CAD build for the part. Positions are in the model's coordinates, mm. A direction names the side the tool comes from. Coordinates: 2 decimals unless noted, no trailing zeros. Loops run counter-clockwise (first coordinate to the right, second up) from the corner with the lowest first, then second, coordinate; pieces in that order, holes last. Notation, with made-up numbers: (-5, -34.75) -> (47, -34.75) arc R32 ccw to (47, -6.75) -> close; hole circle Ø8 at (36.25, -26.5). An arc over 180 degrees is marked (long way). Return JSON: item names as keys, results as strings. Group by question number.
(1) Mould opens along X. For faces 3 (the face through (107.95, -1, 17)), 4 (the face through (-1, -69.85, 17)), 5 (the face through (100.8, -62.9, 27.5)) say: pulls with the +X half, pulls with the -X half, needs draft (parallel to the pull), parting line crosses it, or undercut.
(2) Probe L1, parallel to Y at x = -93.95, z = 18.5; L2, parallel to X at y = -55.85, z = 21; L3, parallel to X at y = 36, z = 9.5. List the from-to ranges inside material, lowest first.
(3) Saw through at C-C on y = 29. Write the cut outline in (x, z), then the cut area to 3 significant figures.
(4) Tool access for faces 1 (the face through (101, 62.7, 27.5)), 2 (the face through (-107.95, 1, 17)): list every direction of +Z, -Z, +X, -X, +Y, -Y with a clear straight run to the whole face (end or side of a thin tool).
(5) Flat gauge pins, fed straight in: pin 1 Ø10 at (x, y) = (-58, 13) entering from +Z; pin 2 Ø4 at (x, y) = (93.95, 55.85) entering from +Z. Where does each tip first touch, or does it go through?
(6) Saw through at A-A on z = 11.5. Write the cut outline in (x, y), then the cut area to 3 significant figures.
(7) Saw through at B-B on x = 24. Write the cut outline in (y, z).
```python
from build123d import *

# Parameters (mm, degrees)
F1_DEPTH  = 30
F2_T      = 10
F5_DEPTH  = 25
F7_W      = 195.9
F7_H      = 119.7
F8_DEPTH  = 5
F9_DEPTH  = 20
F10_D     = 3
F10_DEPTH = 10
F10_TIP   = 0.9012909285
F11_R     = 5


# Not quite as in the source:
# - a shell that OpenCascade refuses in one call is made with other operations: the cavity is built on its own and cut out


with BuildPart() as f1:
    # F0 (on Top) → F1 (new body)
    with BuildSketch(Plane.XY):
        with BuildLine():
            Line((-97.95, -69.85), (97.95, -69.85))
            ThreePointArc((97.95, -69.85), (105.0210678119, -66.9210678119), (107.95, -59.85))
            Line((107.95, -59.85), (107.95, 59.85))
            ThreePointArc((107.95, 59.85), (105.0210678119, 66.9210678119), (97.95, 69.85))
            Line((97.95, 69.85), (-97.95, 69.85))
            ThreePointArc((-97.95, 69.85), (-105.0210678119, 66.9210678119), (-107.95, 59.85))
            Line((-107.95, 59.85), (-107.95, -59.85))
            ThreePointArc((-107.95, -59.85), (-105.0210678119, -66.9210678119), (-97.95, -69.85))
        make_face()
    extrude(amount=F1_DEPTH)

    # F2: shell of thickness 10, made by hand


with BuildPart() as f2_core1:
    # F2_t2: copy of F1
    add(f1.part)

    # the walls: a layer under each face that stays
    f2_faces = [f2_core1.faces().sort_by_distance(p)[0] for p in [
        (0, -69.85, 15),
        (107.95, 0, 15),
        (0, 69.85, 15),
        (-107.95, 0, 15),
        (0, 0, 0),
    ]]
    thicken(f2_faces, amount=-F2_T, mode=Mode.SUBTRACT)


with BuildPart() as f1_1:
    add(f1.part)

    # what is left inside the walls is the cavity
    f2_cavity = [f2_core1.part.solids().sort_by_distance(p)[0] for p in [
        (0, -19.95, 10.1),
    ]]
    add(f2_cavity, mode=Mode.SUBTRACT)

    # F4 (on offset) → F5 (cut)
    with BuildSketch(Plane.XY.offset(25)):
        with BuildLine():
            Line((-95.95, -64.85), (95.95, -64.85))
            ThreePointArc((95.95, -64.85), (100.8997474683, -62.7997474683), (102.95, -57.85))
            Line((102.95, -57.85), (102.95, 57.85))
            ThreePointArc((102.95, 57.85), (100.8997474683, 62.7997474683), (95.95, 64.85))
            Line((95.95, 64.85), (-95.95, 64.85))
            ThreePointArc((-95.95, 64.85), (-100.8997474683, 62.7997474683), (-102.95, 57.85))
            Line((-102.95, 57.85), (-102.95, -57.85))
            ThreePointArc((-102.95, -57.85), (-100.8997474683, -62.7997474683), (-95.95, -64.85))
        make_face()
    extrude(amount=F5_DEPTH, mode=Mode.SUBTRACT)

    # F7 (on face) → F8 (cut)
    with BuildSketch(Plane.XY.offset(10)):
        Rectangle(F7_W, F7_H)
    extrude(amount=-F8_DEPTH, mode=Mode.SUBTRACT)

    # F6 (on face) → F9 (join, through all)
    with BuildSketch(Plane.XY.offset(25)):
        with BuildLine():
            Line((-93.95, 49.85), (-93.95, 55.85))
            Line((-93.95, 55.85), (-87.95, 55.85))
            ThreePointArc((-87.95, 55.85), (-88.3449658462, 57.9909325386), (-89.477864045, 59.85))
            Line((-89.477864045, 59.85), (-97.95, 59.85))
            Line((-97.95, 59.85), (-97.95, 51.377864045))
            ThreePointArc((-97.95, 51.377864045), (-96.0909325386, 50.2449658462), (-93.95, 49.85))
        make_face()
        with BuildLine():
            Line((-87.95, 55.85), (-93.95, 55.85))
            Line((-93.95, 55.85), (-93.95, 49.85))
            ThreePointArc((-93.95, 49.85), (-89.7073593129, 51.6073593129), (-87.95, 55.85))
        make_face()
        with BuildLine():
            Line((93.95, 55.85), (87.95, 55.85))
            ThreePointArc((87.95, 55.85), (89.7073593129, 51.6073593129), (93.95, 49.85))
            Line((93.95, 49.85), (93.95, 55.85))
        make_face()
        with BuildLine():
            ThreePointArc((89.477864045, 59.85), (88.3449658462, 57.9909325386), (87.95, 55.85))
            Line((87.95, 55.85), (93.95, 55.85))
            Line((93.95, 55.85), (93.95, 49.85))
            ThreePointArc((93.95, 49.85), (96.0909325386, 50.2449658462), (97.95, 51.377864045))
            Line((97.95, 51.377864045), (97.95, 59.85))
            Line((97.95, 59.85), (89.477864045, 59.85))
        make_face()
        with BuildLine():
            Line((93.95, -55.85), (93.95, -49.85))
            ThreePointArc((93.95, -49.85), (89.7073593129, -51.6073593129), (87.95, -55.85))
            Line((87.95, -55.85), (93.95, -55.85))
        make_face()
        with BuildLine():
            ThreePointArc((97.95, -51.377864045), (96.0909325386, -50.2449658462), (93.95, -49.85))
            Line((93.95, -49.85), (93.95, -55.85))
            Line((93.95, -55.85), (87.95, -55.85))
            ThreePointArc((87.95, -55.85), (88.3449658462, -57.9909325386), (89.477864045, -59.85))
            Line((89.477864045, -59.85), (97.95, -59.85))
            Line((97.95, -59.85), (97.95, -51.377864045))
        make_face()
        with BuildLine():
            Line((-93.95, -55.85), (-93.95, -49.85))
            ThreePointArc((-93.95, -49.85), (-96.0909325386, -50.2449658462), (-97.95, -51.377864045))
            Line((-97.95, -51.377864045), (-97.95, -59.85))
            Line((-97.95, -59.85), (-89.477864045, -59.85))
            ThreePointArc((-89.477864045, -59.85), (-88.3449658462, -57.9909325386), (-87.95, -55.85))
            Line((-87.95, -55.85), (-93.95, -55.85))
        make_face()
        with BuildLine():
            ThreePointArc((-87.95, -55.85), (-89.7073593129, -51.6073593129), (-93.95, -49.85))
            Line((-93.95, -49.85), (-93.95, -55.85))
            Line((-93.95, -55.85), (-87.95, -55.85))
        make_face()
    extrude(amount=-F9_DEPTH)

    # F10
    with Locations(Plane.XY.offset(25)):
        with Locations((-93.95, 55.85), (-93.95, -55.85), (93.95, -55.85), (93.95, 55.85)):
            Hole(F10_D / 2, depth=F10_DEPTH)
            with Locations((0, 0, -(F10_DEPTH + F10_TIP / 2))):  # 118° drill point
                Cone(0, F10_D / 2, F10_TIP, mode=Mode.SUBTRACT)

    # F11
    f11_edges = [f1_1.edges().sort_by_distance(p)[0] for p in [
        (-107.95, 0, 0),
    ]]
    fillet(f11_edges, radius=F11_R)


solid = f1_1.part
```
Geometry results:
{
 "1": {"face 3": "pulls with the +X half", "face 4": "needs draft", "face 5": "undercut"},
 "2": {"L1": "-69.85 to -57.35, -54.35 to -49.85, 49.85 to 54.35, 57.35 to 69.85", "L2": "-107.95 to -95.45, -92.45 to -87.95, 87.95 to 92.45, 95.45 to 107.95", "L3": "-107.95 to -97.95, 97.95 to 107.95"},
 "3": {"outline": "(-107.95, 5) arc R5 ccw to (-102.95, 0) -> (102.95, 0) arc R5 ccw to (107.95, 5) -> (107.95, 30) -> (102.95, 30) -> (102.95, 25) -> (97.95, 25) -> (97.95, 5) -> (-97.95, 5) -> (-97.95, 25) -> (-102.95, 25) -> (-102.95, 30) -> (-107.95, 30) -> close", "area": "1,520 mm²"},
 "4": {"face 1": "+Z", "face 2": "+Z, -Z, -X, +Y, -Y"},
 "5": {"pin 1": "z = 5", "pin 2": "z = 25"},
 "6": {"outline": "(-107.95, -59.85) arc R10 ccw to (-97.95, -69.85) -> (97.95, -69.85) arc R10 ccw to (107.95, -59.85) -> (107.95, 59.85) arc R10 ccw to (97.95, 69.85) -> (-97.95, 69.85) arc R10 ccw to (-107.95, 59.85) -> close; hole (-97.95, -51.38) arc R6 cw to (-89.48, -59.85) -> (89.48, -59.85) arc R6 cw to (97.95, -51.38) -> (97.95, 51.38) arc R6 cw to (89.48, 59.85) -> (-89.48, 59.85) arc R6 cw to (-97.95, 51.38) -> close", "area": "6,980 mm²"},
 "7": {"outline": "(-69.85, 5) arc R5 ccw to (-64.85, 0) -> (64.85, 0) arc R5 ccw to (69.85, 5) -> (69.85, 30) -> (64.85, 30) -> (64.85, 25) -> (59.85, 25) -> (59.85, 5) -> (-59.85, 5) -> (-59.85, 25) -> (-64.85, 25) -> (-64.85, 30) -> (-69.85, 30) -> close"}
}
